Here's how the part is built. I have some questions about the finished solid (model axes, mm). Face numbers are marked on the shaded views. Round coordinates to 2 decimals unless told otherwise and drop trailing zeros. Order: outer loops, then holes, each group sorted by start corner. A loop starts at its lowest first (then second) coordinate and runs counter-clockwise, first axis right, second up. Notation, with made-up numbers: (60, 22) - (77, 22) arc R23 ccw to (77, 39) - close; hole circle Ø10 at (45, 63). An arc over 180 degrees is marked (long way). One line per item, written item: value.
from build123d import *

# Parameters (mm, degrees)
SKETCH1_W                         = 63.5
SKETCH1_H                         = 38.1
BOSS_EXTRUDE1_DEPTH               = 19.05
F_1_2_0_5025_DIAMETER_HOLE1_D     = 12.7635
F_1_2_0_5025_DIAMETER_HOLE1_DEPTH = 57.144535069
F_1_2_0_5025_DIAMETER_HOLE1_TIP   = 3.834542255
F_35_0_11_DIAMETER_HOLE1_D        = 2.794
F_35_0_11_DIAMETER_HOLE1_DEPTH    = 9.652
F_35_0_11_DIAMETER_HOLE1_TIP      = 0.839402285
F_10_24_TAPPED_HOLE1_D            = 3.7973
F_10_24_TAPPED_HOLE1_DEPTH        = 10.035175986
F_10_24_TAPPED_HOLE1_TIP          = 1.140824014
SKETCH9_R                         = 4.7498
BOSS_EXTRUDE2_DEPTH               = 6.35
F_10_24_TAPPED_HOLE2_D            = 3.7973
F_10_24_TAPPED_HOLE2_DEPTH        = 10.414
F_10_24_TAPPED_HOLE2_CSINK_D      = 5.08
F_10_24_TAPPED_HOLE2_CSINK_ANGLE  = 90
F_10_24_TAPPED_HOLE2_TIP          = 1.140824014
CHAMFER1_SIZE                     = 0.127


with BuildPart() as part:
    # Sketch1 → Boss-Extrude1 (new body)
    with BuildSketch(Plane.XY):
        with Locations((-5.976242834, 24.252126053)):
            Rectangle(SKETCH1_W, SKETCH1_H)
    extrude(amount=BOSS_EXTRUDE1_DEPTH)

    # 1/2 (0.5025) Diameter Hole1
    with Locations(Plane(origin=(25.773757166, 0, 0), x_dir=(0, 0, -1), z_dir=(1, 0, 0))):
        with Locations((-9.525, 24.252126053)):
            Hole(F_1_2_0_5025_DIAMETER_HOLE1_D / 2, depth=F_1_2_0_5025_DIAMETER_HOLE1_DEPTH)
            with Locations((0, 0, -(F_1_2_0_5025_DIAMETER_HOLE1_DEPTH + F_1_2_0_5025_DIAMETER_HOLE1_TIP / 2))):  # 118° drill point
                Cone(0, F_1_2_0_5025_DIAMETER_HOLE1_D / 2, F_1_2_0_5025_DIAMETER_HOLE1_TIP, mode=Mode.SUBTRACT)

    # #35 (0.11) Diameter Hole1
    with Locations(Plane(origin=(0, 0, 0), x_dir=(-1, 0, 0), z_dir=(0, 0, -1))):
        with Locations((26.250138314, 20.873926053), (26.250138314, 27.630326053), (-14.435604522, 27.630326053), (-14.435604522, 20.873926053)):
            Hole(F_35_0_11_DIAMETER_HOLE1_D / 2, depth=F_35_0_11_DIAMETER_HOLE1_DEPTH)
            with Locations((0, 0, -(F_35_0_11_DIAMETER_HOLE1_DEPTH + F_35_0_11_DIAMETER_HOLE1_TIP / 2))):  # 118° drill point
                Cone(0, F_35_0_11_DIAMETER_HOLE1_D / 2, F_35_0_11_DIAMETER_HOLE1_TIP, mode=Mode.SUBTRACT)

    # #10-24 Tapped Hole1
    with Locations(Plane(origin=(25.773757166, 0, 0), x_dir=(0, 0, -1), z_dir=(1, 0, 0))):
        with Locations((-4.7625, 13.478578619), (-14.2875, 35.025673487)):
            Hole(F_10_24_TAPPED_HOLE1_D / 2, depth=F_10_24_TAPPED_HOLE1_DEPTH)
            with Locations((0, 0, -(F_10_24_TAPPED_HOLE1_DEPTH + F_10_24_TAPPED_HOLE1_TIP / 2))):  # 118° drill point
                Cone(0, F_10_24_TAPPED_HOLE1_D / 2, F_10_24_TAPPED_HOLE1_TIP, mode=Mode.SUBTRACT)

    # Sketch9 → Boss-Extrude2 (add)
    with BuildSketch(Plane(origin=(0, 0, 0), x_dir=(-1, 0, 0), z_dir=(0, 0, -1))):
        with Locations((10.738742834, 24.252126053)):
            Circle(SKETCH9_R)
    extrude(amount=BOSS_EXTRUDE2_DEPTH)

    # #10-24 Tapped Hole2
    with Locations(Plane(origin=(0, 0, -6.35), x_dir=(-1, 0, 0), z_dir=(0, 0, -1))):
        with Locations((10.738742834, 24.252126053)):
            CounterSinkHole(F_10_24_TAPPED_HOLE2_D / 2, F_10_24_TAPPED_HOLE2_CSINK_D / 2, depth=F_10_24_TAPPED_HOLE2_DEPTH, counter_sink_angle=F_10_24_TAPPED_HOLE2_CSINK_ANGLE)
            with Locations((0, 0, -(F_10_24_TAPPED_HOLE2_DEPTH + F_10_24_TAPPED_HOLE2_TIP / 2))):  # 118° drill point
                Cone(0, F_10_24_TAPPED_HOLE2_D / 2, F_10_24_TAPPED_HOLE2_TIP, mode=Mode.SUBTRACT)

    # Chamfer1
    chamfer1_edges = [part.edges().sort_by_distance(p)[0] for p in [
        (13.038604522, 20.873926053, 0),
        (13.038604522, 27.630326053, 0),
        (-27.647138314, 27.630326053, 0),
        (-27.647138314, 20.873926053, 0),
        (-37.726242834, 24.252126053, 0),
        (-5.976242834, 43.302126053, 0),
        (-5.988942834, 24.252126053, -6.35),
        (25.773757166, 24.252126053, 0),
        (-5.976242834, 5.202126053, 0),
    ]]
    chamfer(chamfer1_edges, length=CHAMFER1_SIZE)


solid = part.part
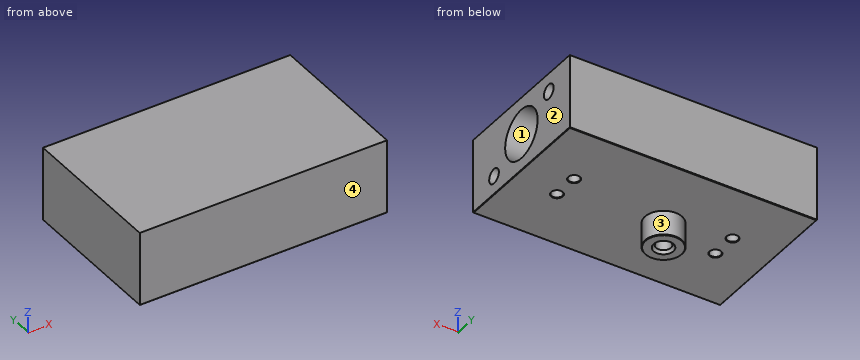
Q1. Will this pin go through, and if not, where does the flat tip stop? pin 1 (2 mm diameter, centred on x = -26.25, y = 27.63, fed in from -Z).
Results list:
pin 1: z = 14.17
Q2. If I drill on line 1 along X through (y, z) = (24.5, 1.5); line 2 along Z through (x, y) = (7.5, 15); line 3 along Z through (x, y) = (-5, 20.5), over which ranges is the centre line in solid material (lowest first)?
Results list:
line 1: -37.73 to -12.62, -8.86 to 25.77
line 2: 0 to 19.05
line 3: 0 to 4.36, 14.69 to 19.05
Q3. If we section it at A-A, the plane y = 17: Please give me the cut outline in (x, z).
Results list:
outline: (-37.73, 0.13) - (-37.6, 0) - (25.65, 0) - (25.77, 0.13) - (25.77, 19.05) - (-37.73, 19.05) - close
Q4. If we section it at C-C, the plane z = -0.75: Please give me the cut outline in (x, y).
Results list:
outline: circle Ø9.5 at (-10.74, 24.25); hole circle Ø3.8 at (-10.74, 24.25)
Q5. We'd pull the mould along Y, two halves only. Please class the marked faces 1, 2, 3 and 4: released by +Y, released by -Y, zero draft, split by the parting line, or undercut.
Results list:
face 1: undercut
face 2: zero draft
face 3: split by the parting line
face 4: released by -Y
